Geometry: see drawing. Coordinates: mm, zero at the bounding-box minimum. A direction names the side the tool comes from. Coordinates: 2 decimals unless noted, no trailing zeros. Loops run counter-clockwise (first coordinate to the right, second up) from the corner with the lowest first, then second, coordinate; pieces in that order, holes last. Notation, with made-up numbers: (75.5, 14.5) - (80.5, 14.5) arc R10 ccw to (80.5, 18.5) - close; hole circle Ø8 at (7.25, 55). An arc over 180 degrees is marked (long way). Use one line per item in the form item = value.
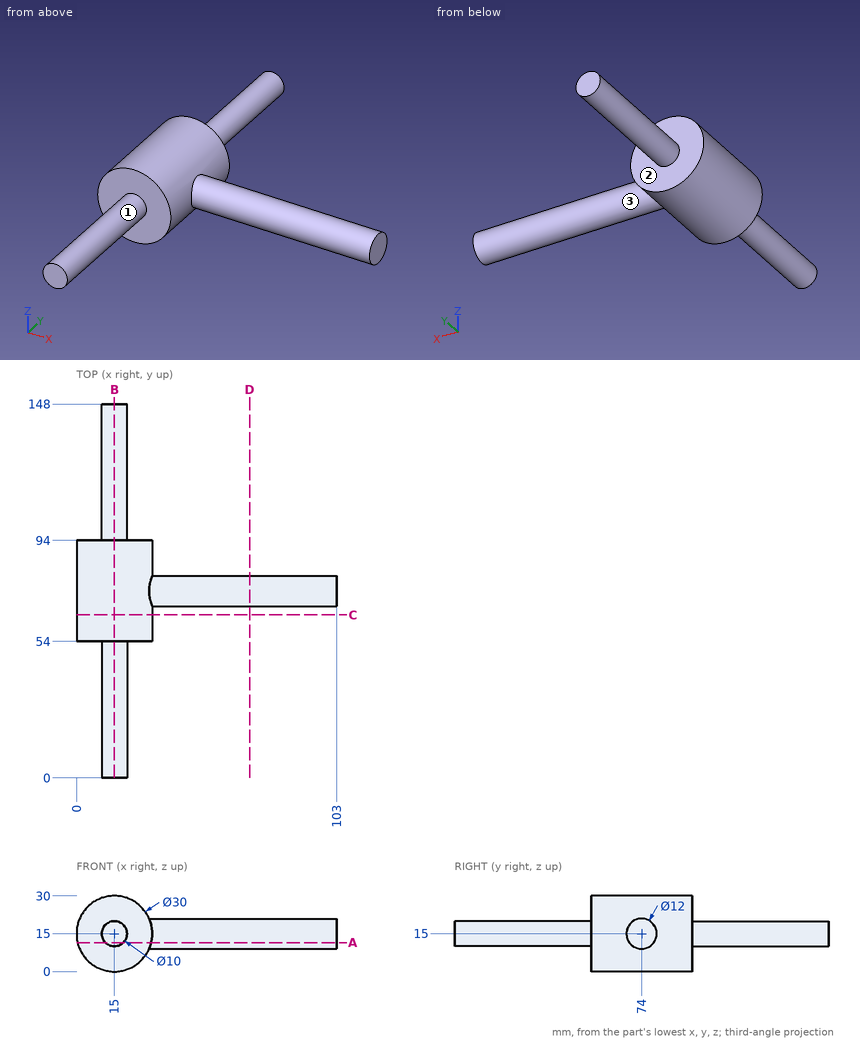
Q1. Cut plane B-B, the plane x = 15. Return loops of the section in (y, z), then the cut area to 3 significant figures.
Check values:
outline = (0, 10) - (54, 10) - (54, 0) - (94, 0) - (94, 10) - (148, 10) - (148, 20) - (94, 20) - (94, 30) - (54, 30) - (54, 20) - (0, 20) - close
area = 2,280 mm²
Q2. Cut plane D-D, the plane x = 68.5. Return loops of the section in (y, z), then the cut area to 3 significant figures.
Check values:
outline = circle Ø12 at (74, 15)
area = 113 mm²
Q3. Cut plane A-A, the plane z = 11.5. Return loops of the section in (x, y).
Check values:
outline = (0.41, 54) - (11.43, 54) - (11.43, 0) - (18.57, 0) - (18.57, 54) - (29.59, 54) - (29.59, 69.13) - (103, 69.13) - (103, 78.87) - (29.59, 78.87) - (29.59, 94) - (18.57, 94) - (18.57, 148) - (11.43, 148) - (11.43, 94) - (0.41, 94) - close
Q4. Set-up query: the marked faces 1, 2 and 3. Return all of +Z, -Z, +X, -X, +Y, -Y with unobstructed straight access to the full face (end or side cutting, diameter ignored); none if empty.
Check values:
face_1 = -Y
face_2 = +Y
face_3 = +X
Q5. Cut plane C-C, the plane y = 64.5. Return loops of the section in (x, z), then the cut area to 3 significant figures.
Check values:
outline = circle Ø30 at (15, 15)
area = 707 mm²
Q6. Ray query, line 1 along Y through (x, z) = (8, 15); line 2 along X through (y, z) = (85.5, 14); line 3 along Y through (x, z) = (43, 13). Return the intervals inside material, ascending. Write a range as [from, to].
Check values:
line_1 = [54, 94]
line_2 = [0.03, 29.97]
line_3 = [68.34, 79.66]
Q7. First-contact query: P1, Ø12, axis at y = 35.5, z = 22.5, coming from the -X side; P2, Ø3, axis at x = 70, y = 71.5, coming from the -Z side; P3, Ø10, axis at y = 68, z = 9.5, coming from the -X side; P4, Ø8, axis at y = 20, z = 26, coming from the -X side. Flat tips, straight axial feed; report the tip coordinate or a pass-through.
Check values:
P1 = 10.23
P2 = 9.08
P3 = 0.01
P4 = through
